from build123d import *

# Parameters (mm, degrees)
F0_R     = 16
F1_DEPTH = 6.6
F2_R     = 3
F3_DEPTH = 2
F4_R     = 1.5
F5_DEPTH = 8.601
F6_R     = 12
F7_DEPTH = 6


with BuildPart() as f1:
    # F0 (on Top) → F1 (new body)
    with BuildSketch(Plane.XY):
        Circle(F0_R)
    extrude(amount=F1_DEPTH)

    # F2 (on face) → F3 (join)
    with BuildSketch(Plane.XY.offset(6.6)):
        Circle(F2_R)
    extrude(amount=F3_DEPTH)

    # F4 (on face) → F5 (cut, through all)
    with BuildSketch(Plane.XY.offset(8.6)):
        Circle(F4_R)
    extrude(amount=-F5_DEPTH, mode=Mode.SUBTRACT)

    # F6 (on face) → F7 (cut)
    with BuildSketch(Plane(origin=(0, 0, 0), x_dir=(1, 0, 0), z_dir=(0, 0, -1))):
        Circle(F6_R)
    extrude(amount=-F7_DEPTH, mode=Mode.SUBTRACT)


solid = f1.part
Geometry: final body of the model. Coordinates: model frame, mm. A direction names the side the tool comes from. Coordinates: 2 decimals unless noted, no trailing zeros. Order: outer loops, then holes, each group sorted by start corner. A loop starts at its lowest first (then second) coordinate and runs counter-clockwise, first axis right, second up.
(1) Access query for faces 1 (the face through (-3.47, -15.62, 3.25)), 2 (the face through (2, 0, 6)). Directions: +Z, -Z, +X, -X, +Y, -Y. A direction counts if a zero-diameter tool reaches every point of the face in a straight line with its end or side. Return the directions, or none.
(2) Section query C-C (z = 1.5). Return the cut outline in (x, y), plus the area to 3 significant figures.
(3) Section query A-A (x = 0). Return the cut outline in (y, z), plus the area to 3 significant figures.
(4) First-contact query: pin 1 (3 mm diameter, centred on x = -12, z = 4, fed in from -Y); pin 2 (1 mm diameter, centred on x = -3.5, y = 4, fed in from +Z); pin 3 (14.5 mm diameter, centred on x = 0, y = 0, fed in from -Z); pin 4 (8 mm diameter, centred on x = 9, y = 9.5, fed in from -Z). Flat tips, straight axial feed; report the tip coordinate or a pass-through.
(5) Draft query along Y for faces 3 (the face through (1.3, -1.3, 8.6)), 4 (the face through (-1.5, 0.07, 7.32)), 5 (the face through (-3, 0, 8)). Return one class per face: pulls with the +Y half, pulls with the -Y half, needs draft (parallel to the pull), parting line crosses it, or undercut.
(6) Material intervals for probe 1 along Y at (x, z) = (0, 7.85); probe 2 along Y at (x, z) = (0, 2.85); probe 3 along X at (y, z) = (-8, 5.5), sorted ascending.
(7) Section query D-D (x = 7). Return the cut outline in (y, z), plus the area to 3 significant figures.
Solution:
1. face 1: +Z, -Z
1. face 2: -Z
2. outline: circle Ø32 at (0, 0); hole circle Ø24 at (0, 0)
2. area: 352 mm2
3. outline: (-16, 0) - (-12, 0) - (-12, 6) - (-1.5, 6) - (-1.5, 8.6) - (-3, 8.6) - (-3, 6.6) - (-16, 6.6) - close; (1.5, 6) - (12, 6) - (12, 0) - (16, 0) - (16, 6.6) - (3, 6.6) - (3, 8.6) - (1.5, 8.6) - close
3. area: 71.4 mm2
4. pin 1: stops at y = -12.07
4. pin 2: stops at z = 6.6
4. pin 3: stops at z = 6
4. pin 4: stops at z = 0
5. face 3: needs draft
5. face 4: undercut
5. face 5: parting line crosses it
6. probe 1: y = -3 to -1.5, 1.5 to 3
6. probe 2: y = -16 to -12, 12 to 16
6. probe 3: x = -13.86 to -8.94, 8.94 to 13.86
7. outline: (-14.39, 0) - (-9.75, 0) - (-9.75, 6) - (9.75, 6) - (9.75, 0) - (14.39, 0) - (14.39, 6.6) - (-14.39, 6.6) - close
7. area: 73.0 mm2
